CAD build for the part. Positions are in the model's coordinates, mm. Give positions to 0.01 mm unless a question says otherwise; leave off trailing zeros. Loops run counter-clockwise (first coordinate to the right, second up) from the corner with the lowest first, then second, coordinate; pieces in that order, holes last. Notation, with made-up numbers: M 59.25,32.25 L 77.25,32.25 A11 cw 77.25,40.25 Z; hole C 84,45 d10. An arc over 180 degrees is marked long. One line per question, with ' | ' between items.
```python
from build123d import *

# Parameters (mm, degrees)
F1_DEPTH = 6.985
F2_DEPTH = 6.985


with BuildPart() as f1:
    # F0 (on Top) → F1 (new body)
    with BuildSketch(Plane.XY):
        with BuildLine():
            Line((0, 15.875), (0, 14.605))
            ThreePointArc((0, 14.605), (2.2450640303, 14.7645517881), (4.445, 15.24))
            ThreePointArc((4.445, 15.24), (2.2450640303, 15.7154482119), (0, 15.875))
        make_face()
        with BuildLine():
            ThreePointArc((-4.445, 15.24), (-2.2450640303, 14.7645517881), (0, 14.605))
            Line((0, 14.605), (0, 15.875))
            ThreePointArc((0, 15.875), (-2.2450640303, 15.7154482119), (-4.445, 15.24))
        make_face()
        with BuildLine():
            Line((0, -15.875), (0, -14.605))
            ThreePointArc((0, -14.605), (-2.2450640303, -14.7645517881), (-4.445, -15.24))
            ThreePointArc((-4.445, -15.24), (-2.2450640303, -15.7154482119), (0, -15.875))
        make_face()
        with BuildLine():
            ThreePointArc((4.445, -15.24), (2.2450640303, -14.7645517881), (0, -14.605))
            Line((0, -14.605), (0, -15.875))
            ThreePointArc((0, -15.875), (2.2450640303, -15.7154482119), (4.445, -15.24))
        make_face()
        with BuildLine():
            ThreePointArc((0, -11.0109), (-11.0109, 0), (0, 11.0109))
            Line((0, 11.0109), (0, 14.605))
            ThreePointArc((0, 14.605), (-2.2450640303, 14.7645517881), (-4.445, 15.24))
            ThreePointArc((-4.445, 15.24), (-7.7179285658, 13.8726062315), (-10.6055411699, 11.8126255123))
            ThreePointArc((-10.6055411699, 11.8126255123), (-15.8737141087, 0.2020529542), (-10.9027768874, -11.5388509455))
            ThreePointArc((-10.9027768874, -11.5388509455), (-10.6764801033, -11.7329434022), (-10.4619588639, -11.9399766219))
            ThreePointArc((-10.4619588639, -11.9399766219), (-7.6339304566, -13.919006099), (-4.445, -15.24))
            ThreePointArc((-4.445, -15.24), (-2.2450640303, -14.7645517881), (0, -14.605))
            Line((0, -14.605), (0, -11.0109))
        make_face()
        with BuildLine():
            ThreePointArc((0, 11.0109), (7.785882057, 7.785882057), (11.0109, 0))
            ThreePointArc((11.0109, 0), (7.785882057, -7.785882057), (0, -11.0109))
            Line((0, -11.0109), (0, -14.605))
            ThreePointArc((0, -14.605), (2.2450640303, -14.7645517881), (4.445, -15.24))
            ThreePointArc((4.445, -15.24), (7.6725040661, -13.897780627), (10.5280263251, -11.8817627774))
            ThreePointArc((10.5280263251, -11.8817627774), (10.7229578197, -11.6931817512), (10.9276762517, -11.5152731942))
            ThreePointArc((10.9276762517, -11.5152731942), (14.5858233483, -6.2665287242), (15.875, 0))
            ThreePointArc((15.875, 0), (14.3832859591, 6.7183859683), (10.188485352, 12.1741690161))
            ThreePointArc((10.188485352, 12.1741690161), (7.4755971863, 14.0046803501), (4.445, 15.24))
            ThreePointArc((4.445, 15.24), (2.2450640303, 14.7645517881), (0, 14.605))
            Line((0, 14.605), (0, 11.0109))
        make_face()
        with BuildLine():
            ThreePointArc((4.445, -15.24), (2.2450640303, -15.7154482119), (0, -15.875))
            ThreePointArc((0, -15.875), (-2.2450640303, -15.7154482119), (-4.445, -15.24))
            ThreePointArc((-4.445, -15.24), (-7.1320670392, -16.2972906415), (-9.5831624007, -17.823830619))
            ThreePointArc((-9.5831624007, -17.823830619), (-7.0669272633, -44.6952792465), (15.875, -30.48))
            ThreePointArc((15.875, -30.48), (14.2580065027, -23.4996794079), (9.7364329992, -17.9413598245))
            ThreePointArc((9.7364329992, -17.9413598245), (7.2182128469, -16.3409396247), (4.445, -15.24))
        make_face()
        with BuildLine():
            ThreePointArc((11.0109, -30.48), (-7.785882057, -38.265882057), (0, -19.4691))
            ThreePointArc((0, -19.4691), (7.785882057, -22.694117943), (11.0109, -30.48))
        make_face(mode=Mode.SUBTRACT)
        with BuildLine():
            ThreePointArc((-4.445, 15.24), (-2.2450640303, 15.7154482119), (0, 15.875))
            ThreePointArc((0, 15.875), (2.2450640303, 15.7154482119), (4.445, 15.24))
            ThreePointArc((4.445, 15.24), (7.4374400281, 16.4550183306), (10.1220432287, 18.2505328867))
            ThreePointArc((10.1220432287, 18.2505328867), (10.7577127256, 18.9684394589), (11.5169632943, 19.5541050033))
            ThreePointArc((11.5169632943, 19.5541050033), (14.7452944578, 24.5985107029), (15.875, 30.48))
            ThreePointArc((15.875, 30.48), (-6.0542794063, 45.1551942362), (-11.2571355427, 19.2865856695))
            ThreePointArc((-11.2571355427, 19.2865856695), (-10.8608812375, 18.9498902987), (-10.5011212887, 18.574451853))
            ThreePointArc((-10.5011212887, 18.574451853), (-7.6567798508, 16.5735501541), (-4.445, 15.24))
        make_face()
        with BuildLine():
            ThreePointArc((11.0109, 30.48), (7.785882057, 22.694117943), (0, 19.4691))
            ThreePointArc((0, 19.4691), (-7.785882057, 38.265882057), (11.0109, 30.48))
        make_face(mode=Mode.SUBTRACT)
    extrude(amount=F1_DEPTH)

    # F0 (on Top) → F2 (join)
    with BuildSketch(Plane.XY):
        with BuildLine():
            ThreePointArc((0, 11.0109), (7.785882057, 7.785882057), (11.0109, 0))
            ThreePointArc((11.0109, 0), (7.785882057, -7.785882057), (0, -11.0109))
            Line((0, -11.0109), (0, -14.605))
            ThreePointArc((0, -14.605), (2.2450640303, -14.7645517881), (4.445, -15.24))
            ThreePointArc((4.445, -15.24), (7.6725040661, -13.897780627), (10.5280263251, -11.8817627774))
            ThreePointArc((10.5280263251, -11.8817627774), (10.7229578197, -11.6931817512), (10.9276762517, -11.5152731942))
            ThreePointArc((10.9276762517, -11.5152731942), (14.5858233483, -6.2665287242), (15.875, 0))
            ThreePointArc((15.875, 0), (14.3832859591, 6.7183859683), (10.188485352, 12.1741690161))
            ThreePointArc((10.188485352, 12.1741690161), (7.4755971863, 14.0046803501), (4.445, 15.24))
            ThreePointArc((4.445, 15.24), (2.2450640303, 14.7645517881), (0, 14.605))
            Line((0, 14.605), (0, 11.0109))
        make_face()
        with BuildLine():
            ThreePointArc((0, -11.0109), (-11.0109, 0), (0, 11.0109))
            Line((0, 11.0109), (0, 14.605))
            ThreePointArc((0, 14.605), (-2.2450640303, 14.7645517881), (-4.445, 15.24))
            ThreePointArc((-4.445, 15.24), (-7.7179285658, 13.8726062315), (-10.6055411699, 11.8126255123))
            ThreePointArc((-10.6055411699, 11.8126255123), (-15.8737141087, 0.2020529542), (-10.9027768874, -11.5388509455))
            ThreePointArc((-10.9027768874, -11.5388509455), (-10.6764801033, -11.7329434022), (-10.4619588639, -11.9399766219))
            ThreePointArc((-10.4619588639, -11.9399766219), (-7.6339304566, -13.919006099), (-4.445, -15.24))
            ThreePointArc((-4.445, -15.24), (-2.2450640303, -14.7645517881), (0, -14.605))
            Line((0, -14.605), (0, -11.0109))
        make_face()
        with BuildLine():
            ThreePointArc((-4.445, 15.24), (-2.2450640303, 15.7154482119), (0, 15.875))
            ThreePointArc((0, 15.875), (2.2450640303, 15.7154482119), (4.445, 15.24))
            ThreePointArc((4.445, 15.24), (7.4374400281, 16.4550183306), (10.1220432287, 18.2505328867))
            ThreePointArc((10.1220432287, 18.2505328867), (10.7577127256, 18.9684394589), (11.5169632943, 19.5541050033))
            ThreePointArc((11.5169632943, 19.5541050033), (14.7452944578, 24.5985107029), (15.875, 30.48))
            ThreePointArc((15.875, 30.48), (-6.0542794063, 45.1551942362), (-11.2571355427, 19.2865856695))
            ThreePointArc((-11.2571355427, 19.2865856695), (-10.8608812375, 18.9498902987), (-10.5011212887, 18.574451853))
            ThreePointArc((-10.5011212887, 18.574451853), (-7.6567798508, 16.5735501541), (-4.445, 15.24))
        make_face()
        with BuildLine():
            ThreePointArc((11.0109, 30.48), (7.785882057, 22.694117943), (0, 19.4691))
            ThreePointArc((0, 19.4691), (-7.785882057, 38.265882057), (11.0109, 30.48))
        make_face(mode=Mode.SUBTRACT)
        with BuildLine():
            ThreePointArc((-10.6055411699, 11.8126255123), (-7.7179285658, 13.8726062315), (-4.445, 15.24))
            ThreePointArc((-4.445, 15.24), (-7.6567798508, 16.5735501541), (-10.5011212887, 18.574451853))
            ThreePointArc((-10.5011212887, 18.574451853), (-9.2646720581, 15.1736384914), (-10.6055411699, 11.8126255123))
        make_face()
        with BuildLine():
            ThreePointArc((10.1220432287, 18.2505328867), (7.4374400281, 16.4550183306), (4.445, 15.24))
            ThreePointArc((4.445, 15.24), (7.4755971863, 14.0046803501), (10.188485352, 12.1741690161))
            ThreePointArc((10.188485352, 12.1741690161), (9.1465341041, 15.2013209708), (10.1220432287, 18.2505328867))
        make_face()
        with BuildLine():
            ThreePointArc((4.445, -15.24), (2.2450640303, -15.7154482119), (0, -15.875))
            ThreePointArc((0, -15.875), (-2.2450640303, -15.7154482119), (-4.445, -15.24))
            ThreePointArc((-4.445, -15.24), (-7.1320670392, -16.2972906415), (-9.5831624007, -17.823830619))
            ThreePointArc((-9.5831624007, -17.823830619), (-7.0669272633, -44.6952792465), (15.875, -30.48))
            ThreePointArc((15.875, -30.48), (14.2580065027, -23.4996794079), (9.7364329992, -17.9413598245))
            ThreePointArc((9.7364329992, -17.9413598245), (7.2182128469, -16.3409396247), (4.445, -15.24))
        make_face()
        with BuildLine():
            ThreePointArc((11.0109, -30.48), (-7.785882057, -38.265882057), (0, -19.4691))
            ThreePointArc((0, -19.4691), (7.785882057, -22.694117943), (11.0109, -30.48))
        make_face(mode=Mode.SUBTRACT)
        with BuildLine():
            ThreePointArc((10.5280263251, -11.8817627774), (7.6725040661, -13.897780627), (4.445, -15.24))
            ThreePointArc((4.445, -15.24), (7.2182128469, -16.3409396247), (9.7364329992, -17.9413598245))
            ThreePointArc((9.7364329992, -17.9413598245), (9.119170131, -14.7792206259), (10.5280263251, -11.8817627774))
        make_face()
        with BuildLine():
            ThreePointArc((-9.5831624007, -17.823830619), (-7.1320670392, -16.2972906415), (-4.445, -15.24))
            ThreePointArc((-4.445, -15.24), (-7.6339304566, -13.919006099), (-10.4619588639, -11.9399766219))
            ThreePointArc((-10.4619588639, -11.9399766219), (-9.0711708687, -14.7398066276), (-9.5831624007, -17.823830619))
        make_face()
        with BuildLine():
            ThreePointArc((-11.2571355427, 19.2865856695), (-10.8849537771, 18.9243344514), (-10.5011212887, 18.574451853))
            ThreePointArc((-10.5011212887, 18.574451853), (-10.8608812375, 18.9498902987), (-11.2571355427, 19.2865856695))
        make_face()
        with BuildLine():
            ThreePointArc((11.5169632943, 19.5541050033), (10.7577127256, 18.9684394589), (10.1220432287, 18.2505328867))
            ThreePointArc((10.1220432287, 18.2505328867), (10.8391178558, 18.881329856), (11.5169632943, 19.5541050033))
        make_face()
        with BuildLine():
            ThreePointArc((10.9276762517, -11.5152731942), (10.7229578197, -11.6931817512), (10.5280263251, -11.8817627774))
            ThreePointArc((10.5280263251, -11.8817627774), (10.7294161966, -11.7002244885), (10.9276762517, -11.5152731942))
        make_face()
        with BuildLine():
            ThreePointArc((-10.9027768874, -11.5388509455), (-10.6842505064, -11.7414827052), (-10.4619588639, -11.9399766219))
            ThreePointArc((-10.4619588639, -11.9399766219), (-10.6764801033, -11.7329434022), (-10.9027768874, -11.5388509455))
        make_face()
    extrude(amount=F2_DEPTH)


solid = f1.part
```
Item 1: Saw through at A-A on y = -22.5. Give the cut face in (x, z) (3 decimals), and give its area (3 significant figures).
Conclusion:
outline: M -13.724,0 L -7.587,0 L -7.587,6.985 L -13.724,6.985 Z; M 7.587,0 L 13.724,0 L 13.724,6.985 L 7.587,6.985 Z | area: 85.7 mm²
Item 2: Saw through at B-B on z = 2.5. Give the cut face in (x, y) (3 decimals).
Conclusion:
outline: M -10.606,11.813 A15.875 ccw -10.462,-11.94 A5.08 cw -9.583,-17.824 A15.875 ccw long 9.736,-17.941 A5.08 cw 10.528,-11.882 A15.875 ccw 10.188,12.174 A5.08 cw 10.122,18.251 A15.875 ccw long -10.501,18.574 A5.08 cw Z; hole C 0,-30.48 d22.022; hole C 0,0 d22.022; hole C 0,30.48 d22.022
Item 3: Drop flat-ended pins along their axis: P1, Ø1.5, axis at x = -1.5, z = 3, coming from the -Y side; P2, Ø13, axis at x = 0, y = 30.48, coming from the +Z side; P3, Ø3, axis at y = -2, z = 1.5, coming from the -X side; P4, Ø2, axis at x = -6.5, z = 1, coming from the +Y side. Give the stop position or say it passes through.
Conclusion:
P1: y = -46.34 | P2: through | P3: x = -15.87 | P4: y = 45.37
Item 4: Saw through at C-C on y = -5. Give the cut face in (x, z) (3 decimals), and give its area (3 significant figures).
Conclusion:
outline: M -15.067,0 L -9.81,0 L -9.81,6.985 L -15.067,6.985 Z; M 9.81,0 L 15.067,0 L 15.067,6.985 L 9.81,6.985 Z | area: 73.4 mm²
Item 5: Drill centre lines: line 1 along Y through (x, z) = (-12, 4); line 2 along X through (y, z) = (-30.48, 1.75) (3 decimals); line 3 along Y through (x, z) = (-14, 2). Where is each one in solid material? Low to high. Write a range as [from, to].
Conclusion:
line 1: [-40.87, -20.09], [-10.39, 10.39], [20.09, 40.87] | line 2: [-15.875, -11.011], [11.011, 15.875] | line 3: [-37.96, -23], [-7.48, 7.48], [23, 37.96]
